```python
from build123d import *

# Parameters (mm, degrees)
SKETCH1_W           = 106.32
SKETCH1_H           = 66
SKETCH1_R           = 2
SKETCH1_W_2         = 12.8
SKETCH1_H_2         = 12.8
BOSS_EXTRUDE1_DEPTH = 6
SKETCH4_R           = 1.75
CUT_EXTRUDE1_DEPTH  = 67.939412158


with BuildPart() as part:
    # Sketch1 → Boss-Extrude1 (new body)
    with BuildSketch(Plane(origin=(0, 0, 0), x_dir=(1, 0, 0), z_dir=(0, 1, 0))):
        with Locations((-4.77, 0)):
            Rectangle(SKETCH1_W, SKETCH1_H)
        with Locations(Location((20.152543264, -20.152543264, 0), (0, 0, 270))):
            Circle(SKETCH1_R, mode=Mode.SUBTRACT)
        with Locations(Location((20.152543264, 20.152543264, 0), (0, 0, 270))):
            Circle(SKETCH1_R, mode=Mode.SUBTRACT)
        with Locations(Location((-20.152543264, -20.152543264, 0), (0, 0, 270))):
            Circle(SKETCH1_R, mode=Mode.SUBTRACT)
        with Locations(Location((-20.152543264, 20.152543264, 0), (0, 0, 270))):
            Circle(SKETCH1_R, mode=Mode.SUBTRACT)
        Rectangle(SKETCH1_W_2, SKETCH1_H_2, mode=Mode.SUBTRACT)
    extrude(amount=BOSS_EXTRUDE1_DEPTH)

    # Sketch4 → Cut-Extrude1 (cut, through all)
    with BuildSketch(Plane(origin=(0, 6, 0), x_dir=(1, 0, 0), z_dir=(0, 1, 0))):
        with Locations(Location((-50.93, 20, 0), (0, 0, 270))):
            Circle(SKETCH4_R)
        with Locations(Location((-44.93, -20, 0), (0, 0, 270))):
            Circle(SKETCH4_R)
        with Locations(Location((35.39, -20, 0), (0, 0, 270))):
            Circle(SKETCH4_R)
        with Locations(Location((35.39, 20, 0), (0, 0, 270))):
            Circle(SKETCH4_R)
    extrude(amount=-CUT_EXTRUDE1_DEPTH, mode=Mode.SUBTRACT)


solid = part.part
```
The model under review builds one solid part; all positions refer to its coordinate system, in mm. A direction names the side the tool comes from. Round coordinates to 2 decimals unless told otherwise and drop trailing zeros. Order: outer loops, then holes, each group sorted by start corner. A loop starts at its lowest first (then second) coordinate and runs counter-clockwise, first axis right, second up.
(1) Take a section at C-C, the plane x = 35.39. State the section outline as (y, z) points, plus the area to 3 significant figures.
Working result:
outline: (0, -33) - (6, -33) - (6, -21.75) - (0, -21.75) - close; (0, -18.25) - (6, -18.25) - (6, 18.25) - (0, 18.25) - close; (0, 21.75) - (6, 21.75) - (6, 33) - (0, 33) - close
area: 354 mm2
(2) For P1, Ø6, axis at x = -22.5, z = -5, coming from the -Y side, flat-tipped, find the tip position at first contact; note if it passes through.
Working result:
P1: stops at y = 0
(3) Mouldability with a two-part tool opening along Z and no side actions: class faces 1 (the face through (-6, 3, -33)), 2 (the face through (0, 3, -6.4)), 3 (the face through (-6, 0, -8)) as released by +Z, released by -Z, zero draft, split by the parting line, or undercut.
Working result:
face 1: released by -Z
face 2: undercut
face 3: zero draft
(4) Tool access review of faces 4 (the face through (-6, 6, -8)), 5 (the face through (-6.4, 3, 0)): name each direction out of +Z, -Z, +X, -X, +Y, -Y from which nothing blocks a thin tool from reaching the whole face with its end or side.
Working result:
face 4: +Z, -Z, +X, -X, +Y
face 5: +Y, -Y
(5) Take a section at B-B, the plane x = -4. State the section outline as (y, z) points, plus the area to 3 significant figures.
Working result:
outline: (0, -33) - (6, -33) - (6, -6.4) - (0, -6.4) - close; (0, 6.4) - (6, 6.4) - (6, 33) - (0, 33) - close
area: 319 mm2
(6) Wall thickness on L1, parallel to X at y = 4.7, z = -20; L2, parallel to X at y = 4, z = 20; L3, parallel to Z at x = 5, y = 4.2: over which ranges is each line inside the solid? List them lowest first.
Working result:
L1: x = -57.93 to -52.68, -49.18 to -22.15, -18.16 to 18.16, 22.15 to 33.64, 37.14 to 48.39
L2: x = -57.93 to -46.68, -43.18 to -22.15, -18.16 to 18.16, 22.15 to 33.64, 37.14 to 48.39
L3: z = -33 to -6.4, 6.4 to 33
(7) Take a section at A-A, the plane z = 4.5. State the section outline as (x, y) points.
Working result:
outline: (-57.93, 0) - (-6.4, 0) - (-6.4, 6) - (-57.93, 6) - close; (6.4, 0) - (48.39, 0) - (48.39, 6) - (6.4, 6) - close
(8) Take a section at D-D, the plane z = -20. State the section outline as (x, y) points.
Working result:
outline: (-57.93, 0) - (-52.68, 0) - (-52.68, 6) - (-57.93, 6) - close; (-49.18, 0) - (-22.15, 0) - (-22.15, 6) - (-49.18, 6) - close; (-18.16, 0) - (18.16, 0) - (18.16, 6) - (-18.16, 6) - close; (22.15, 0) - (33.64, 0) - (33.64, 6) - (22.15, 6) - close; (37.14, 0) - (48.39, 0) - (48.39, 6) - (37.14, 6) - close
